Read the model definition and answer for the solid it produces. Units are mm, in the model's axes. Face numbers are marked on the shaded views. Give positions to 0.01 mm unless a question says otherwise; leave off trailing zeros. Order: outer loops, then holes, each group sorted by start corner. A loop starts at its lowest first (then second) coordinate and runs counter-clockwise, first axis right, second up. Notation, with made-up numbers: (69, -38) - (73, -38) arc R27 cw to (73, -14) - close; hole circle Ø5 at (-4, -18.75). An arc over 180 degrees is marked (long way). Return JSON: item names as keys, results as strings.
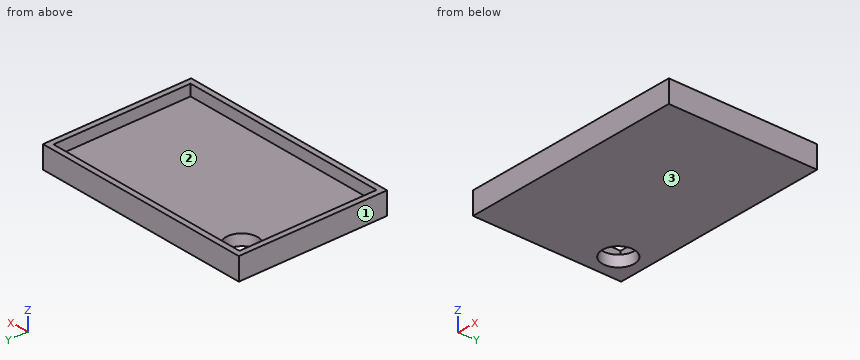
```python
from build123d import *

# Parameters (mm, degrees)
F0_W     = 60
F0_H     = 40
F1_DEPTH = 3
F2_W     = 57
F2_H     = 37
F3_DEPTH = 3
F6_R     = 4.2845281604
F7_DEPTH = 6


# Not quite as in the source:
# - the program builds the solid bodies; features that only make, move or delete a surface that nothing else refers to are left out


with BuildPart() as f1:
    # F0 (on Top) → F1 (new body, symmetric)
    with BuildSketch(Plane.XY):
        Rectangle(F0_W, F0_H)
    extrude(amount=F1_DEPTH, both=True)

    # F2 (on face) → F3 (cut)
    with BuildSketch(Plane.XY.offset(3)):
        Rectangle(F2_W, F2_H)
    extrude(amount=-F3_DEPTH, mode=Mode.SUBTRACT)

    # F6 (on face) → F7 (cut)
    with BuildSketch(Plane.XY):
        with Locations((-22.8839740157, 12.9562756047)):
            Circle(F6_R)
    extrude(amount=-F7_DEPTH, mode=Mode.SUBTRACT)


solid = f1.part
```
Q1. A cutting plane is placed at B-B (y = 11.5). Write down the section's boundary in (x, z), and give its area (3 significant figures).
Values:
{"outline": "(-30, -3) - (-26.91, -3) - (-26.91, 0) - (-28.5, 0) - (-28.5, 3) - (-30, 3) - close; (-18.85, -3) - (30, -3) - (30, 3) - (28.5, 3) - (28.5, 0) - (-18.85, 0) - close", "area": "165 mm²"}
Q2. A cutting plane is placed at A-A (z = 2.4). Write down the section's boundary in (x, y), and give its area (3 significant figures).
Values:
{"outline": "(-30, -20) - (30, -20) - (30, 20) - (-30, 20) - close; hole (-28.5, -18.5) - (28.5, -18.5) - (28.5, 18.5) - (-28.5, 18.5) - close", "area": "291 mm²"}
Q3. Consider L1, parallel to X at y = 15.5, z = 0.65; L2, parallel to Y at x = -21, z = 2.5; L3, parallel to Z at x = 27, y = 4. Determine where each line is inside the solid, lowest interval first.
Values:
{"L1": "x = -30 to -28.5, 28.5 to 30", "L2": "y = -20 to -18.5, 18.5 to 20", "L3": "z = -3 to 0"}
Q4. A cutting plane is placed at C-C (x = 23.5). Write down the section's boundary in (y, z), and give its area (3 significant figures).
Values:
{"outline": "(-20, -3) - (20, -3) - (20, 3) - (18.5, 3) - (18.5, 0) - (-18.5, 0) - (-18.5, 3) - (-20, 3) - close", "area": "129 mm²"}
Q5. A cutting plane is placed at D-D (x = -23). Write down the section's boundary in (y, z), and give its area (3 significant figures).
Values:
{"outline": "(-20, -3) - (8.67, -3) - (8.67, 0) - (-18.5, 0) - (-18.5, 3) - (-20, 3) - close; (17.24, -3) - (20, -3) - (20, 3) - (18.5, 3) - (18.5, 0) - (17.24, 0) - close", "area": "103 mm²"}
Q6. Determine the mould class of the marked faces 1, 2 and 3 for opening direction X: released by +X, released by -X, zero draft, split by the parting line, or undercut.
Values:
{"face 1": "released by -X", "face 2": "undercut", "face 3": "zero draft"}
Q7. Given pin 1 (1 mm diameter, centred on x = -3.5, y = 11.5, fed in from +Z), flat-ended and moving along its own axis, determine where the tip first touches the part or whether it passes through.
Values:
{"pin 1": "stops at z = 0"}
